Source: CAD feature listing. Evaluate the final solid. Frame: model axes, mm. A direction names the side the tool comes from. Give positions to 0.01 mm unless a question says otherwise; leave off trailing zeros. Order: outer loops, then holes, each group sorted by start corner. A loop starts at its lowest first (then second) coordinate and runs counter-clockwise, first axis right, second up. Notation, with made-up numbers: (0, 33) - (51, 33) arc R8 ccw to (51, 43) - close; hole circle Ø10 at (67.5, 16). An arc over 180 degrees is marked (long way). Write each question's results on one line, items separated by ' | '. Start each with the question number.
Item 1: Section B-B on x = 0. Output: boundary loops of the cut face in (y, z), and give its area (3 significant figures).
Item 2: Set-up query: faces 5 (the cylindrical face through (-0.09, -9.95, 0.99)), 6 (the flat face through (-27, 85, -18)). Return all of +Z, -Z, +X, -X, +Y, -Y with unobstructed straight access to the full face (end or side cutting, diameter ignored); none if empty.
Item 3: Contact query for flat-ended pins moving along their axis: pin 1 Ø5.5 at (x, y) = (10.39, -6) entering from -Z; pin 2 Ø3.5 at (x, y) = (-10.39, 6) entering from +Z; pin 3 Ø1 at (y, z) = (55.5, 0.5) entering from +X; pin 4 Ø0.5 at (x, z) = (24.5, 1) entering from -Y. Output: stop coordinate, or through.
Item 4: Section D-D on y = 0. Output: boundary loops of the cut face in (x, z), and give its area (3 significant figures).
Item 5: Mould query, pull axis Z, two halves, no side actions, for faces 1 (the cylindrical face through (-28.014, 98.414, -23.292)), 2 (the flat face through (28, 60, -15)), 3 (the cylindrical face through (-28.014, 78.414, -23.292)), 4 (the flat face through (0, 61, 0)). Classes: released by +Z, released by -Z, zero draft, split by the parting line, or undercut.
Item 6: Section C-C on z = -27.5. Output: boundary loops of the cut face in (x, y), and give its area (3 significant figures).
Item 7: Section A-A on y = 100. Output: boundary loops of the cut face in (x, z), and give its area (3 significant figures).
Item 8: Line query: line 1 along Y through (x, z) = (28.35, -23.5); line 2 along X through (y, z) = (86, -16); line 3 along X through (y, z) = (-12, 1.35). Output: solid intervals per line, ascending.
Autodesk Inventor part; units mm, degrees
ref_plane "YZ Plane" through (0, 0, 0) normal (1, 0, 0) x (0, 1, 0)
ref_plane "XZ Plane" through (0, 0, 0) normal (0, 1, 0) x (-1, 0, 0)
ref_plane "XY Plane" through (0, 0, 0) normal (0, 0, 1) x (1, 0, 0)
sketch "スケッチ1" plane through (0, 0, 0) normal (0, 0, 1) x (1, 0, 0)
  circle A0 centre (0, 0) radius 18.5
  line L0 (0, 0) -> (0, 60)
  line L1 (0, 60) -> (25, 60)
  line L2 (25, 60) -> (25, 110)
  line L3 (25, 110) -> (0, 110)
  line L4 (0, 110) -> (0, 60)
  line L5 (25, 60) -> (18.3958, -1.9608)
  line L6 (0, 60) -> (-25, 60)
  line L7 (-25, 60) -> (-25, 110)
  line L8 (-25, 110) -> (0, 110)
  line L9 (-25, 60) -> (-18.3958, -1.9608)
  point P0 (-18.3958, -1.9608)
  dimension "d0" = 37
  dimension "d1" = 60
  dimension "d2" = 50
  dimension "d3" = 25
extrude "プレート1" add sketch "スケッチ1" along normal blind 2
sketch "スケッチ2" plane through (27, 60, -2) normal (1, 0, 0) x (0, 1, 0)
  line L0 (50, 0) -> (0, 0)
  line L1 (0, 0) -> (0, -31.5)
  line L2 (0, -31.5) -> (50, -31.5)
  line L3 (50, -31.5) -> (50, 0)
edge flange "フランジ1" height 35.5 angle 90 thickness 2 bend radius 2 thickness toward (1, 0, 0) relief tear relief width 2 relief depth 1 edges at (25, 85, 0) wall of the first edge with corners at (27, 110, -2) (27, 60, -2) (27, 60, -33.5) (27, 110, -33.5)
bend "曲げ1"
corner "コーナー1"
sketch "スケッチ3" plane through (-27, 110, -2) normal (-1, 0, 0) x (0, -1, 0)
  line L0 (50, 0) -> (0, 0)
  line L1 (0, 0) -> (0, -31.5)
  line L2 (0, -31.5) -> (50, -31.5)
  line L3 (50, -31.5) -> (50, 0)
edge flange "フランジ2" height 35.5 angle 90 thickness 2 bend radius 2 thickness toward (-1, 0, 0) relief tear relief width 2 relief depth 1 edges at (-25, 85, 0) wall of the first edge with corners at (-27, 60, -2) (-27, 110, -2) (-27, 110, -33.5) (-27, 60, -33.5)
bend "曲げ2"
corner "コーナー2"
sketch "スケッチ4" plane through (0, 0, 2) normal (0, 0, 1) x (1, 0, 0)
  circle A0 centre (0, 0) radius 7
  dimension "d25" = 14
extrude "押し出し1" cut sketch "スケッチ4" against normal blind 10
sketch "スケッチ5" plane through (0, 0, 2) normal (0, 0, 1) x (1, 0, 0)
  circle A0 centre (0, 0) radius 12
  point P0 (0, 12)
  point P1 (-10.3923, 6)
  point P2 (-10.3923, -6)
  point P3 (0, -12)
  point P4 (10.3923, -6)
  point P5 (10.3923, 6)
  dimension "d28" = 24
  dimension "d31" = 360
hole "穴1" at (0, 12, 2) at (-10.3923, 6, 2) at (-10.3923, -6, 2) at (0, -12, 2) at (10.3923, -6, 2) at (10.3923, 6, 2) direction (0, 0, -1) diameter 4.1 end through all
sketch "スケッチ6" plane through (29, 60, -33.5) normal (1, 0, 0) x (0, 0, -1)
  line L0 (0, 0) -> (0, 50)
  line L1 (0, 10) -> (-31.5, 10)
  line L2 (-31.5, 50) -> (-31.5, 0)
  line L3 (0, 0) -> (-31.5, 0)
  line L4 (0, 50) -> (-31.5, 50)
  line L5 (-10, 50) -> (-10, 10)
  point P0 (-33.5, -60)
  point P1 (-10, 20)
  point P2 (-10, 40)
  point P3 (-33.5, 50)
  dimension "d40" = 10
  dimension "d42" = 10
  dimension "d43" = 20
  dimension "d62" = 23.5
hole "穴2" at (29, 80, -23.5) at (29, 100, -23.5) direction (-1, 0, 0) diameter 3.2 end through all
sketch "スケッチ7" plane through (0, 0, 2) normal (0, 0, 1) x (1, 0, 0)
  line L0 (-15, 100) -> (15, 100)
  line L1 (15, 100) -> (15, 60)
  line L2 (15, 60) -> (-15, 60)
  line L3 (-15, 60) -> (-15, 100)
  line L4 (-25, 110) -> (25, 110)
  line L5 (-25, 60) -> (-25, 110)
  line L6 (25, 110) -> (25, 60)
  circle A0 centre (0, 0) radius 7
  circle A1 centre (0, 0) radius 8.5
  line L7 (-8.4521, -0.9009) -> (-13.8775, 50)
  line L8 (-18.3958, -1.9608) -> (-25, 60)
  line L9 (8.4521, -0.9009) -> (13.8775, 50)
  line L10 (25, 60) -> (18.3958, -1.9608)
  line L11 (-13.8775, 50) -> (13.8775, 50)
  line L12 (-10.6799, 20) -> (10.6799, 20)
  dimension "d51" = 10
  dimension "d52" = 10
  dimension "d53" = 10
  dimension "d54" = 40
  dimension "d55" = 10
  dimension "d56" = 10
  dimension "d57" = 20
extrude "押し出し2" [suppressed]
fillet "フィレット1" [suppressed]
fillet "フィレット2" radius 2 4 edges at (-28, 60, -33.5) (-28, 110, -33.5) (28, 60, -33.5) (28, 110, -33.5)
sketch "スケッチ8" plane through (0, 0, 2) normal (0, 0, 1) x (1, 0, 0)
  line L0 (-25, 110) -> (-25, 60)
  line L1 (-25, 60) -> (25, 60)
  line L2 (25, 60) -> (25, 50)
  line L3 (25, 50) -> (-25, 50)
  line L4 (-25, 50) -> (-25, 60)
  point P0 (0, 0)
  dimension "d63" = 10
extrude "押し出し3" add sketch "スケッチ8" against normal blind 2
equation "\"d38\" = Thickness"
equation "\"d4\" = Thickness"
equation "\"d5\" = BendReliefWidth"
equation "\"d6\" = BendReliefDepth"
equation "\"d7\" = MinimumRemnant"
equation "\"d8\" = TransitionRadius"
equation "\"d11\" = BendRadius"
equation "\"d12\" = CornerReliefSize"
equation "\"d13\" = GapSize"
equation "\"d14\" = JacobiRadiusSize"
equation "\"d15\" = BendReliefWidth"
equation "\"d16\" = BendReliefDepth"
equation "\"d17\" = MinimumRemnant"
equation "\"d18\" = TransitionRadius"
equation "\"d21\" = BendRadius"
equation "\"d22\" = CornerReliefSize"
equation "\"d23\" = GapSize"
equation "\"d24\" = JacobiRadiusSize"
equation "\"BendRadius\" = Thickness"
equation "\"BendReliefWidth\" = Thickness"
equation "\"BendReliefDepth\" = 0.5 * Thickness"
equation "\"CornerReliefSize\" = 4 * Thickness"
equation "\"MinimumRemnant\" = 2 * Thickness"
equation "\"TransitionRadius\" = BendRadius"
equation "\"JacobiRadiusSize\" = BendRadius"
equation "\"GapSize\" = Thickness"
properties part number "servoplate1_forR6" material "アルミニウム 6061"
Evaluation:
1) outline: (-18.5, 0) - (-14.05, 0) - (-14.05, 2) - (-18.5, 2) - close; (-9.95, 0) - (-7, 0) - (-7, 2) - (-9.95, 2) - close; (7, 0) - (9.95, 0) - (9.95, 2) - (7, 2) - close; (14.05, 0) - (110, 0) - (110, 2) - (14.05, 2) - close | area: 213 mm^2
2) face 5: +Z, -Z | face 6: -Z, +Y, -Y
3) pin 1: stops at z = 0 | pin 2: passes through | pin 3: stops at x = 25 | pin 4: stops at y = 50
4) outline: (-18.6, 0) - (-7, 0) - (-7, 2) - (-18.6, 2) - close; (7, 0) - (18.6, 0) - (18.6, 2) - (7, 2) - close | area: 46.4 mm^2
5) face 1: undercut | face 2: zero draft | face 3: undercut | face 4: released by -Z
6) outline: (-29, 60) - (-27, 60) - (-27, 110) - (-29, 110) - close; (27, 60) - (29, 60) - (29, 110) - (27, 110) - close | area: 200 mm^2
7) outline: (-29, -33.5) - (-27, -33.5) - (-27, -25.1) - (-29, -25.1) - close; (-29, -21.9) - (-27, -21.9) - (-27, -2) arc R2 cw to (-25, 0) - (25, 0) arc R2 cw to (27, -2) - (27, -21.9) - (29, -21.9) - (29, -2) arc R4 ccw to (25, 2) - (-25, 2) arc R4 ccw to (-29, -2) - close; (27, -33.5) - (29, -33.5) - (29, -25.1) - (27, -25.1) - close | area: 232 mm^2
8) line 1: y = 60 to 78.4, 81.6 to 98.4, 101.6 to 110 | line 2: x = -29 to -27, 27 to 29 | line 3: x = -14.08 to -2.05, 2.05 to 14.08
